Check sheet for the modelled part. Datum: model origin and axes. Units: mm. A direction names the side the tool comes from. Give positions to 0.01 mm unless a question says otherwise; leave off trailing zeros. Order: outer loops, then holes, each group sorted by start corner. A loop starts at its lowest first (then second) coordinate and runs counter-clockwise, first axis right, second up.
Item 1: Release check for a two-part mould opening along Y. For faces 1 (the flat face through (20, 24.13, 1)), 2 (the flat face through (40.64, 12, 1)), 3 (the flat face through (41.2, 17.891, 3.1)) record: released by +Y, released by -Y, zero draft, split by the parting line, or undercut.
Item 2: Access from +Z, -Z, +X, -X, +Y, -Y to the whole of each face (thin tool, end or side, straight path). Record for faces 4 (the flat face through (41.2, 11.181, 3.1)), 5 (the flat face through (29, 4.799, 2)), 6 (the flat face through (31.375, 7, 2)), 7 (the flat face through (9, 20, 2)).
Item 3: Material ranges on line 1 along Y through (x, z) = (2, 0.4); line 2 along X through (y, z) = (22.13, 0.85); line 3 along X through (y, z) = (2.13, 0.35), recorded low to high.
Item 4: Sectioned sample at B-B on y = 22.13. Record the boundary of the cut face in (x, z).
Item 5: Gauge pin test, flat ends, axial feed: P1, Ø0.8, axis at x = 42, z = 3, coming from the -Y side; P2, Ø0.7, axis at x = 40, y = 6, coming from the -Z side; P3, Ø0.8, axis at x = 41, z = 3, coming from the +Y side; P4, Ø1.2, axis at x = 27.5, y = 6.5, coming from the +Z side. Record the tip position at first contact, or that the pin passes through.
Item 6: Sectioned sample at C-C on x = 11.5. Record the boundary of the cut face in (y, z).
Item 7: Sectioned sample at D-D on y = 10. Record the boundary of the cut face in (x, z), and give its area (3 significant figures).
Item 8: Sectioned sample at A-A on z = 0.85. Record the boundary of the cut face in (x, y), and give its area (3 significant figures).
from build123d import *

# Parameters (mm, degrees)
SKETCH1_W           = 40.64
SKETCH1_H           = 24.13
BOSS_EXTRUDE1_DEPTH = 1.6
SKETCH2_W           = 13.99999994
SKETCH2_H           = 16
BOSS_EXTRUDE2_DEPTH = 2.5
SKETCH3_R           = 1.1
CUT_EXTRUDE1_DEPTH  = 2.5
LPATTERN1_COUNT     = 2
LPATTERN1_PITCH     = 36.5
LPATTERN2_COUNT     = 2
LPATTERN2_PITCH     = 20
SKETCH4_R           = 1.1
CUT_EXTRUDE2_DEPTH  = 2.5
BOSS_EXTRUDE3_DEPTH = 2.5
SKETCH6_W           = 0.64
SKETCH6_H           = 0.64
BOSS_EXTRUDE4_DEPTH = 1
SKETCH8_W           = 0.635
SKETCH8_H           = 0.64
BOSS_EXTRUDE5_DEPTH = 8
LPATTERN7_COUNT     = 6
LPATTERN7_PITCH     = 2.45
SKETCH9_W           = 3.5
SKETCH9_H           = 6.5
BOSS_EXTRUDE6_DEPTH = 1.5
SKETCH10_W          = 5
SKETCH10_H          = 4
BOSS_EXTRUDE7_DEPTH = 1.5


with BuildPart() as part:
    # Sketch1 → Boss-Extrude1 (new body)
    with BuildSketch(Plane.XY):
        with Locations((20.32, 12.065)):
            Rectangle(SKETCH1_W, SKETCH1_H)
    extrude(amount=BOSS_EXTRUDE1_DEPTH)

    # Sketch2 → Boss-Extrude2 (add)
    with BuildSketch(Plane.XY):
        with Locations((8.99999997, 12)):
            Rectangle(SKETCH2_W, SKETCH2_H)
    extrude(amount=BOSS_EXTRUDE2_DEPTH)

    # Sketch3 → Cut-Extrude1 (cut)
    with BuildSketch(Plane.XY):
        with Locations(Location((2, 22.129999936, 0), (0, 0, 180))):
            Circle(SKETCH3_R)
    cut_extrude1 = extrude(amount=CUT_EXTRUDE1_DEPTH, mode=Mode.SUBTRACT)

    # LPattern1: Cut-Extrude1 ×2
    with Locations(*[(i * LPATTERN1_PITCH, 0, 0) for i in range(1, LPATTERN1_COUNT)]):
        add(cut_extrude1, mode=Mode.SUBTRACT)

    # LPattern2: Cut-Extrude1 ×2
    with Locations(*[(0, -i * LPATTERN2_PITCH, 0) for i in range(1, LPATTERN2_COUNT)]):
        add(cut_extrude1, mode=Mode.SUBTRACT)

    # Sketch4 → Cut-Extrude2 (cut)
    with BuildSketch(Plane.XY.offset(1.6)):
        with Locations((38.64, 2.000000064)):
            Circle(SKETCH4_R)
    extrude(amount=-CUT_EXTRUDE2_DEPTH, mode=Mode.SUBTRACT)

    # Sketch5 → Boss-Extrude3 (add)
    with BuildSketch(Plane.XY):
        with BuildLine():
            Line((35.249253939, 18.555999972), (35.249253939, 5.556000064))
            ThreePointArc((35.249253939, 5.556000064), (37.249254003, 3.556), (39.249254067, 5.556000064))
            Line((39.249254067, 5.556000064), (39.249254067, 18.555999972))
            ThreePointArc((39.249254067, 18.555999972), (37.249254003, 20.556000036), (35.249253939, 18.555999972))
        make_face()
    extrude(amount=BOSS_EXTRUDE3_DEPTH)

    # Sketch6 → Boss-Extrude4 (add)
    with BuildSketch(Plane.XY.offset(2.5)):
        with Locations((37.220253939, 18.210599972)):
            Rectangle(SKETCH6_W, SKETCH6_H)
    boss_extrude4 = extrude(amount=BOSS_EXTRUDE4_DEPTH)

    # Sketch8 → Boss-Extrude5 (add)
    with BuildSketch(Plane(origin=(37.540253939, 0, 0), x_dir=(0, 0, -1), z_dir=(1, 0, 0))):
        with Locations((-3.1825, 18.210599972)):
            Rectangle(SKETCH8_W, SKETCH8_H)
    boss_extrude5 = extrude(amount=BOSS_EXTRUDE5_DEPTH)

    # LPattern7: Boss-Extrude4, Boss-Extrude5 ×6
    with Locations(*[(0, -i * LPATTERN7_PITCH, 0) for i in range(1, LPATTERN7_COUNT)]):
        add(boss_extrude4)
        add(boss_extrude5)

    # Sketch9 → Boss-Extrude6 (add)
    with BuildSketch(Plane.XY.offset(1.6)):
        with Locations((26.068319719, 19.356)):
            Rectangle(SKETCH9_W, SKETCH9_H)
    extrude(amount=BOSS_EXTRUDE6_DEPTH)

    # Sketch10 → Boss-Extrude7 (add)
    with BuildSketch(Plane.XY.offset(1.6)):
        with Locations((28.874727699, 6.798621882)):
            Rectangle(SKETCH10_W, SKETCH10_H)
    extrude(amount=BOSS_EXTRUDE7_DEPTH)


solid = part.part
Report:
1. face 1: released by +Y
1. face 2: zero draft
1. face 3: undercut
2. face 4: +Z, +X, -X
2. face 5: +Z, -Y
2. face 6: +Z, +Y, -Y
2. face 7: +Z, -X, +Y
3. line 1: y = 0 to 1.03, 3.23 to 21.03, 23.23 to 24.13
3. line 2: x = 0 to 0.9, 3.1 to 37.4, 39.6 to 40.64
3. line 3: x = 0 to 0.9, 3.1 to 37.55, 39.73 to 40.64
4. outline: (0, 0) - (0.9, 0) - (0.9, 1.6) - (0, 1.6) - close; (3.1, 0) - (37.4, 0) - (37.4, 1.6) - (27.82, 1.6) - (27.82, 3.1) - (24.32, 3.1) - (24.32, 1.6) - (3.1, 1.6) - close; (39.6, 0) - (40.64, 0) - (40.64, 1.6) - (39.6, 1.6) - close
5. P1: stops at y = 5.64
5. P2: stops at z = 0
5. P3: stops at y = 18.53
5. P4: stops at z = 3.1
6. outline: (0, 0) - (24.13, 0) - (24.13, 1.6) - (20, 1.6) - (20, 2.5) - (4, 2.5) - (4, 1.6) - (0, 1.6) - close
7. outline: (0, 0) - (40.64, 0) - (40.64, 1.6) - (39.25, 1.6) - (39.25, 2.5) - (35.25, 2.5) - (35.25, 1.6) - (16, 1.6) - (16, 2.5) - (2, 2.5) - (2, 1.6) - (0, 1.6) - close
7. area: 81.2 mm2
8. outline: (0, 0) - (40.64, 0) - (40.64, 24.13) - (0, 24.13) - close; hole circle Ø2.2 at (2, 2.13); hole circle Ø2.2 at (2, 22.13); hole circle Ø2.2 at (38.5, 22.13); hole circle Ø2.2 at (38.64, 2)
8. area: 965 mm2
